Can you work these out from the model? Positions are in its coordinate system, mm. Give positions to 0.01 mm unless a question says otherwise; leave off trailing zeros. Write each loop counter-clockwise with the first axis right and the second up, starting at its lowest first coordinate (ties: lowest second). Pieces come first, ordered by that corner, then holes. Notation, with made-up numbers: (-0.5, 22.5) - (14.5, 22.5) arc R23 ccw to (14.5, 45.5) - close; hole circle Ø3 at (69.5, 65). An arc over 180 degrees is marked (long way). Use a Markdown table: item, result. Add a question column.
```python
from build123d import *

# Parameters (mm, degrees)
RESSALTO_EXTRUS_O1_DEPTH = 5
FURO_COM_FOLGA_DE_M51_D  = 5.5


with BuildPart() as part:
    # Esboço1 → Ressalto-extrusão1 (new body)
    with BuildSketch(Plane.XY):
        Polygon((0, 0), (0, 34.5), (108, 73), (108, 53), (118, 53), (118, 0), align=None)
    extrude(amount=RESSALTO_EXTRUS_O1_DEPTH)

    # Furo com folga de M51 (through all)
    with Locations(Plane.XY.offset(5)):
        with Locations((100, 6), (70, 6), (40, 6)):
            Hole(FURO_COM_FOLGA_DE_M51_D / 2)


solid = part.part
```
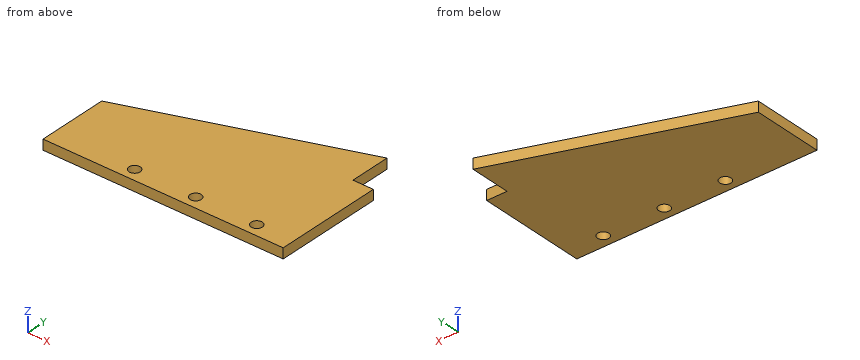
Q1. I'm going to push flat-ended pins straight in: P1, Ø4.5, axis at x = 40, y = 6, coming from the +Z side; P2, Ø2.5, axis at x = 111.5, z = 3, coming from the +Y side; P3, Ø1, axis at x = 80.5, z = 4.5, coming from the +Y side (3 decimals); P4, Ø1.5, axis at y = 63, z = 1, coming from the +X side. Where does each tip first touch, or does it pass through?
Q2. Suppose I cut it at A-A (y = 6). Please give me the cut outline in (x, z).
Q3. Suppose I cut it at C-C (x = 100). Please give me the cut outline in (y, z).
Q4. Suppose I cut it at B-B (z = 3.6). Please give me the cut outline in (x, y).
Q5. Suppose I cut it at D-D (x = 40). Please give me the cut outline in (y, z), and give its area (3 significant figures).
Q6. If I drill on probe 1 along X at (y, z) = (4, 1.35); probe 2 along Y at (x, z) = (100, 3.2); probe 3 along Y at (x, z) = (70, 2.7), over which ranges is the centre line in solid material (lowest first)? Write a range as [from, to].
Derived:
| question | item | result |
|---|---|---|
| 1 | P1 | through |
| 1 | P2 | y = 53 |
| 1 | P3 | y = 63.375 |
| 1 | P4 | x = 108 |
| 2 | outline | (0, 0) - (37.25, 0) - (37.25, 5) - (0, 5) - close; (42.75, 0) - (67.25, 0) - (67.25, 5) - (42.75, 5) - close; (72.75, 0) - (97.25, 0) - (97.25, 5) - (72.75, 5) - close; (102.75, 0) - (118, 0) - (118, 5) - (102.75, 5) - close |
| 3 | outline | (0, 0) - (3.25, 0) - (3.25, 5) - (0, 5) - close; (8.75, 0) - (70.15, 0) - (70.15, 5) - (8.75, 5) - close |
| 4 | outline | (0, 0) - (118, 0) - (118, 53) - (108, 53) - (108, 73) - (0, 34.5) - close; hole circle Ø5.5 at (40, 6); hole circle Ø5.5 at (70, 6); hole circle Ø5.5 at (100, 6) |
| 5 | outline | (0, 0) - (3.25, 0) - (3.25, 5) - (0, 5) - close; (8.75, 0) - (48.76, 0) - (48.76, 5) - (8.75, 5) - close |
| 5 | area | 216 mm² |
| 6 | probe 1 | [0, 38.11], [41.89, 68.11], [71.89, 98.11], [101.89, 118] |
| 6 | probe 2 | [0, 3.25], [8.75, 70.15] |
| 6 | probe 3 | [0, 3.25], [8.75, 59.45] |
